The model under review builds one solid part; all positions refer to its coordinate system, in mm. Round coordinates to 2 decimals unless told otherwise and drop trailing zeros. Write each loop counter-clockwise with the first axis right and the second up, starting at its lowest first coordinate (ties: lowest second). Pieces come first, ordered by that corner, then holes. Notation, with made-up numbers: (86, 51) -> (120, 51) arc R29 cw to (120, 79) -> close; hole circle Ø6 at (-2, 56.5). An arc over 180 degrees is marked (long way). Return JSON: item names as keys, results as strings. Group by question number.
1. For line 1 along Y through (x, z) = (-8.5, 0.55); line 2 along Y through (x, z) = (14.5, 0.45); line 3 along Z through (x, y) = (20, 2.5), list the stretches that pass through material, from the lowest coordinate up. Write a range as from..to.
2. Take a section at A-A, the plane x = -4. Write out the cut boundary in (y, z), then the cut area to 3 significant figures.
3. Clearance check with flat-ended pins moving along their axes: P1, Ø1, axis at y = -17, z = 1, coming from the -X side; P2, Ø2, axis at x = 6, y = 17.5, coming from the +Z side; P3, Ø1.5, axis at x = 20, z = 2.5, coming from the +Y side. State where each tip first meets the part, or that it passes through.
from build123d import *

# Parameters (mm, degrees)
SKETCH_R              = 29
PAD_DEPTH             = 3
POCKET_DEPTH          = 5
POLARPATTERN_COUNT    = 2
POCKET001_DEPTH       = 5
POLARPATTERN001_COUNT = 2
SKETCH003_R           = 18
POCKET002_DEPTH       = 2.4
SKETCH004_R           = 17
POCKET003_DEPTH       = 5
POCKET004_DEPTH       = 1.5
POLARPATTERN002_COUNT = 2
PAD001_DEPTH          = 1.6
POLARPATTERN003_COUNT = 2
SKETCH007_R           = 18.340375
PAD002_DEPTH          = 0.4
SKETCH008_R           = 17
POCKET005_DEPTH       = 5


with BuildPart() as part:
    # Sketch → Pad (new body)
    with BuildSketch(Plane.XY):
        Circle(SKETCH_R)
    extrude(amount=PAD_DEPTH)

    # Sketch001 (on Face3 of Pad) → Pocket (cut)
    with BuildSketch(Plane.XY.offset(3)):
        with BuildLine():
            ThreePointArc((-18.385067, -15.426903), (-10.142838, -21.751387), (0, -24))
            ThreePointArc((1.989789, -29.812024), (3.071599, -26.195037), (0, -24))
            ThreePointArc((1.989789, -29.812024), (2.178472, -31.958585), (3.600531, -30.339612))
            ThreePointArc((3.600531, -30.339612), (4.313448, -25.265566), (0, -22.5))
            ThreePointArc((-17.236, -14.462721), (-9.508911, -20.391925), (0, -22.5))
            ThreePointArc((-17.236, -14.462721), (-18.296812, -14.365288), (-18.385067, -15.426903))
        make_face()
    pocket = extrude(amount=-POCKET_DEPTH, mode=Mode.SUBTRACT)

    # PolarPattern: Pocket ×2 about axis
    polarpattern_axis = Axis((0, 0, 3), (0, 0, 1))
    for i in range(1, POLARPATTERN_COUNT):
        add(pocket.rotate(polarpattern_axis, i * 360 / POLARPATTERN_COUNT), mode=Mode.SUBTRACT)

    # Sketch002 (on Face4 of PolarPattern) → Pocket001 (cut)
    with BuildSketch(Plane.XY.offset(3)):
        with BuildLine():
            add(Edge.make_bspline(
                [(-3.074709, 28.315083), (-42.734669, 12.512014), (-16.852234, -23.673746)],
                knots=[0, 0, 0, 1, 1, 1], degree=2))
            Line((-16.852234, -23.673746), (-19.979143, -30.365301))
            Line((-19.979143, -30.365301), (-32.54401, -28.825899))
            Line((-32.54401, -28.825899), (-39.32571, 4.3753))
            Line((-39.32571, 4.3753), (-7.235262, 36.220139))
            Line((-7.235262, 36.220139), (-3.074709, 28.315083))
        make_face()
    pocket001 = extrude(amount=-POCKET001_DEPTH, mode=Mode.SUBTRACT)

    # PolarPattern001: Pocket001 ×2 about axis
    polarpattern001_axis = Axis((0, 0, 3), (0, 0, 1))
    for i in range(1, POLARPATTERN001_COUNT):
        add(pocket001.rotate(polarpattern001_axis, i * 360 / POLARPATTERN001_COUNT), mode=Mode.SUBTRACT)

    # Sketch003 (on Face4 of PolarPattern001) → Pocket002 (cut)
    with BuildSketch(Plane.XY.offset(3)):
        Circle(SKETCH003_R)
    extrude(amount=-POCKET002_DEPTH, mode=Mode.SUBTRACT)

    # Sketch004 (on Face18 of Pocket002) → Pocket003 (cut)
    with BuildSketch(Plane.XY.offset(0.6)):
        Circle(SKETCH004_R)
    extrude(amount=-POCKET003_DEPTH, mode=Mode.SUBTRACT)

    # Sketch005 (on Face4 of Pocket003) → Pocket004 (cut)
    with BuildSketch(Plane.XY.offset(3)):
        Polygon((-7.733806, -22.017185), (-1.653993, -23.383749), (2.389916, -24.108864), (3.923815, -27.065102), (3.45663, -30.749018), (-4.573239, -30.749018), (-10.02356, -30.749018), align=None)
    pocket004 = extrude(amount=-POCKET004_DEPTH, mode=Mode.SUBTRACT)

    # PolarPattern002: Pocket004 ×2 about axis
    polarpattern002_axis = Axis((0, 0, 3), (0, 0, 1))
    for i in range(1, POLARPATTERN002_COUNT):
        add(pocket004.rotate(polarpattern002_axis, i * 360 / POLARPATTERN002_COUNT), mode=Mode.SUBTRACT)

    # Sketch006 (on Face28 of PolarPattern002) → Pad001 (join)
    with BuildSketch(Plane.XY.offset(1.5)):
        with BuildLine():
            ThreePointArc((-7.90278, -22.661555), (-4.00766, -23.663023), (0, -24))
            ThreePointArc((3.010027, -25.819366), (1.758576, -24.49018), (0, -24))
            ThreePointArc((-8.410088, -24.596145), (-2.768435, -25.846386), (3.010027, -25.819366))
            Line((-7.90278, -22.661555), (-8.410088, -24.596145))
        make_face()
    pad001 = extrude(amount=PAD001_DEPTH)

    # PolarPattern003: Pad001 ×2 about axis
    polarpattern003_axis = Axis((0, 0, 1.5), (0, 0, 1))
    for i in range(1, POLARPATTERN003_COUNT):
        add(pad001.rotate(polarpattern003_axis, i * 360 / POLARPATTERN003_COUNT))

    # Sketch007 (on Face6 of PolarPattern003) → Pad002 (join)
    with BuildSketch(Plane.XY.offset(3)):
        Circle(SKETCH007_R)
    extrude(amount=-PAD002_DEPTH)

    # Sketch008 (on Face35 of Pad002) → Pocket005 (cut)
    with BuildSketch(Plane.XY.offset(3)):
        Circle(SKETCH008_R)
    extrude(amount=-POCKET005_DEPTH, mode=Mode.SUBTRACT)


solid = part.part
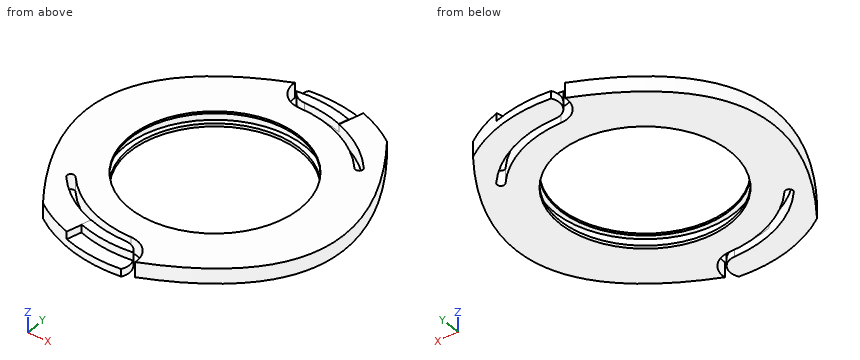
Output:
{
 "1": {"line 1": "y = -27.73..-22.44, -20.83..-14.72, 14.72..25.91", "line 2": "y = -22.46..-8.87, 8.87..17.2, 19.12..25.11", "line 3": "z = 0..3"},
 "2": {"outline": "(-28.72, 0) -> (-23.66, 0) -> (-23.66, 3.1) -> (-25.68, 3.1) -> (-25.68, 1.5) -> (-28.72, 1.5) -> close; (-22.14, 0) -> (-16.52, 0) -> (-16.52, 0.6) -> (-17.55, 0.6) -> (-17.55, 2.6) -> (-16.52, 2.6) -> (-16.52, 3) -> (-22.14, 3) -> close; (16.52, 0) -> (24.69, 0) -> (24.69, 3) -> (16.52, 3) -> (16.52, 2.6) -> (17.55, 2.6) -> (17.55, 0.6) -> (16.52, 0.6) -> close", "area": "48.1 mm^2"},
 "3": {"P1": "stops at x = -21.45", "P2": "stops at z = 3", "P3": "stops at y = 20.15"}
}
